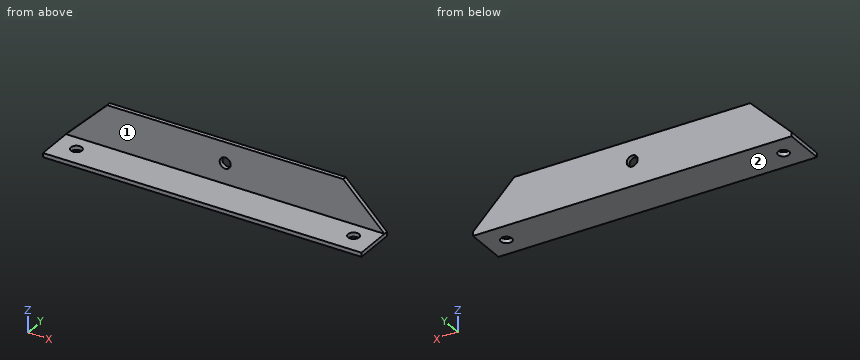
```python
from build123d import *

# Parameters (mm, degrees)
SKETCH1_W                = 231.4
SKETCH1_H                = 30
BOSS_EXTRUDE1_DEPTH      = 3
BOSS_EXTRUDE2_DEPTH      = 3
F_8_0_8_DIAMETER_HOLE2_D = 8
F_8_0_8_DIAMETER_HOLE1_D = 8


with BuildPart() as part:
    # Sketch1 → Boss-Extrude1 (new body)
    with BuildSketch(Plane.XY):
        with Locations((0, -15)):
            Rectangle(SKETCH1_W, SKETCH1_H)
    extrude(amount=BOSS_EXTRUDE1_DEPTH)

    # Sketch3 → Boss-Extrude2 (add)
    with BuildSketch(Plane(origin=(0, 0, 0), x_dir=(1, 0, 0), z_dir=(0, 1, 0))):
        Polygon((-85.7, -33), (85.7, -33), (115.7, -3), (-115.7, -3), align=None)
    extrude(amount=-BOSS_EXTRUDE2_DEPTH)

    # Ø8.0 (8) Diameter Hole2 (through all)
    with Locations(Plane(origin=(0, 0, 0), x_dir=(-1, 0, 0), z_dir=(0, 0, -1))):
        with Locations((100.7, -15), (-100.7, -15)):
            Hole(F_8_0_8_DIAMETER_HOLE2_D / 2)

    # Ø8.0 (8) Diameter Hole1 (through all)
    with Locations(Plane(origin=(0, -3, 0), x_dir=(-1, 0, 0), z_dir=(0, -1, 0))):
        with Locations((0, -18)):
            Hole(F_8_0_8_DIAMETER_HOLE1_D / 2)


solid = part.part
```
Read the model definition and answer for the solid it produces. Units are mm, in the model's axes. Face numbers are marked on the shaded views. A direction names the side the tool comes from. Round coordinates to 2 decimals unless told otherwise and drop trailing zeros. Write each loop counter-clockwise with the first axis right and the second up, starting at its lowest first coordinate (ties: lowest second). Pieces come first, ordered by that corner, then holes. Notation, with made-up numbers: (-39.75, -23.75) -> (-33.75, -23.75) arc R22 ccw to (-33.75, 3.25) -> close; hole circle Ø4 at (18, 81.5). An arc over 180 degrees is marked (long way). Answer in a Markdown table with one row per item. Add a question column.
1) Find section C-C, the plane z = 18. Determine the outline of the cut face in (x, y), and give its area (3 significant figures).
2) Find section B-B, the plane y = -15. Determine the outline of the cut face in (x, z), and give its area (3 significant figures).
3) Consider line 1 (Z direction, x = 0, y = -1.9); line 2 (Y direction, x = -100.7, z = 0.8); line 3 (Z direction, x = 76, y = -21.5). Determine where each line is inside the solid, lowest interval first.
4) Given P1, Ø6, axis at x = 41.5, z = 26.5, coming from the -Y side; P2, Ø13, axis at x = -100.7, y = -15, coming from the +Z side, each flat-ended and moving along its own axis, determine where each tip first touches the part or whether it passes through.
5) Find section A-A, the plane x = -100.7. Determine the outline of the cut face in (y, z).
6) Find section D-D, the plane x = -71. Determine the outline of the cut face in (y, z).
7) Which of the six approach directions +Z, -Z, +X, -X, +Y, -Y give full straight-line access (tool end or side, diameter ignored) to the marked faces 1 and 2?
Findings below:
| question | item | result |
|---|---|---|
| 1 | outline | (-100.7, -3) -> (-4, -3) -> (-4, 0) -> (-100.7, 0) -> close; (4, -3) -> (100.7, -3) -> (100.7, 0) -> (4, 0) -> close |
| 1 | area | 580 mm² |
| 2 | outline | (-115.7, 0) -> (-104.7, 0) -> (-104.7, 3) -> (-115.7, 3) -> close; (-96.7, 0) -> (96.7, 0) -> (96.7, 3) -> (-96.7, 3) -> close; (104.7, 0) -> (115.7, 0) -> (115.7, 3) -> (104.7, 3) -> close |
| 2 | area | 646 mm² |
| 3 | line 1 | 0 to 14, 22 to 33 |
| 3 | line 2 | -30 to -19, -11 to 0 |
| 3 | line 3 | 0 to 3 |
| 4 | P1 | y = -3 |
| 4 | P2 | z = 3 |
| 5 | outline | (-30, 0) -> (-19, 0) -> (-19, 3) -> (-30, 3) -> close; (-11, 0) -> (0, 0) -> (0, 18) -> (-3, 18) -> (-3, 3) -> (-11, 3) -> close |
| 6 | outline | (-30, 0) -> (0, 0) -> (0, 33) -> (-3, 33) -> (-3, 3) -> (-30, 3) -> close |
| 7 | face 1 | +Z, +X, -X, -Y |
| 7 | face 2 | -Z, +X, -X, +Y, -Y |
